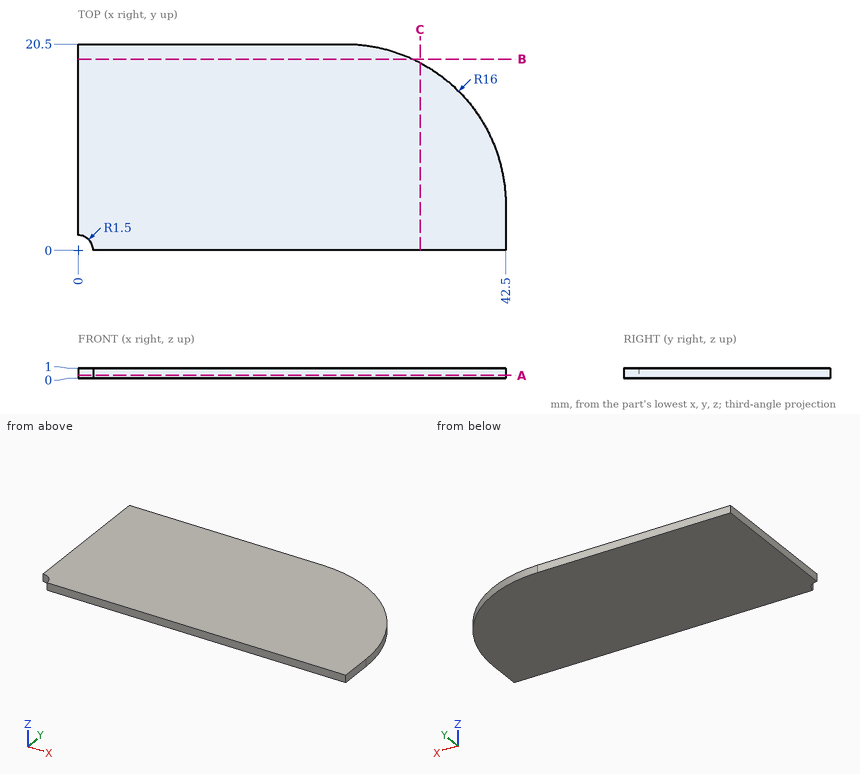
Source: three-view drawing plus pictorial views. Frame: mm from the lowest corner of the part. Give positions to 0.01 mm unless a question says otherwise; leave off trailing zeros. Order: outer loops, then holes, each group sorted by start corner. A loop starts at its lowest first (then second) coordinate and runs counter-clockwise, first axis right, second up. Notation, with made-up numbers: (58, -18) - (92, -18) arc R12 ccw to (92, 5) - close; hole circle Ø6 at (9, -16.75). An arc over 180 degrees is marked (long way). Answer as a JSON object with one key per item and string values. Group by question number.
Q1. Cut plane B-B, the plane y = 19. Output: boundary loops of the cut face in (x, z).
Q2. Line query: probe 1 along X at (y, z) = (5.75, 0.35); probe 2 along X at (y, z) = (8.25, 0.4); probe 3 along Y at (x, z) = (33, 0.8). Output: solid intervals per line, ascending.
Q3. Cut plane C-C, the plane x = 34. Output: boundary loops of the cut face in (y, z).
Q4. Cut plane A-A, the plane z = 0.3. Output: boundary loops of the cut face in (x, y), then the cut area to 3 significant figures.
Results:
{
 "1": {"outline": "(0, 0) - (33.26, 0) - (33.26, 1) - (0, 1) - close"},
 "2": {"probe 1": "0 to 42.45", "probe 2": "0 to 42.05", "probe 3": "0 to 19.12"},
 "3": {"outline": "(0, 0) - (18.63, 0) - (18.63, 1) - (0, 1) - close"},
 "4": {"outline": "(0, 1.5) arc R1.5 cw to (1.5, 0) - (42.5, 0) - (42.5, 4.5) arc R16 ccw to (26.5, 20.5) - (0, 20.5) - close", "area": "815 mm^2"}
}
